from build123d import *

# Parameters (mm, degrees)
SKETCH1_R           = 15
BOSS_EXTRUDE1_DEPTH = 50
SKETCH2_R           = 1.5
BOSS_EXTRUDE2_DEPTH = 15
BOSS_EXTRUDE4_DEPTH = 3
SKETCH5_W           = 34
SKETCH5_H           = 3
BOSS_EXTRUDE5_DEPTH = 40
FILLET2_R           = 2
SKETCH6_R           = 30
BOSS_EXTRUDE6_DEPTH = 7
CUT_EXTRUDE1_DEPTH  = 7
SKETCH8_R           = 5
BOSS_EXTRUDE7_DEPTH = 5
SKETCH9_R           = 1.5
CUT_EXTRUDE2_DEPTH  = 5


with BuildPart() as part:
    # Sketch1 → Boss-Extrude1 (new body)
    with BuildSketch(Plane.XY):
        Circle(SKETCH1_R)
    extrude(amount=BOSS_EXTRUDE1_DEPTH)

    # Sketch2 → Boss-Extrude2 (add)
    with BuildSketch(Plane.XY.offset(50)):
        Circle(SKETCH2_R)
    extrude(amount=BOSS_EXTRUDE2_DEPTH)

    # Sketch4 → Boss-Extrude4 (add)
    with BuildSketch(Plane.XY.offset(50)):
        with BuildLine():
            Line((-17, 0), (-17, 30))
            Line((-17, 30), (17, 30))
            Line((17, 30), (17, 0))
            ThreePointArc((17, 0), (0, -17), (-17, 0))
        make_face()
    extrude(amount=BOSS_EXTRUDE4_DEPTH)

    # Sketch5 → Boss-Extrude5 (add)
    with BuildSketch(Plane(origin=(0, 0, 50), x_dir=(-1, 0, 0), z_dir=(0, 0, -1))):
        with Locations((0, 28.5)):
            Rectangle(SKETCH5_W, SKETCH5_H)
    extrude(amount=BOSS_EXTRUDE5_DEPTH)

    # Fillet2
    fillet2_edges = [part.edges().sort_by_distance(p)[0] for p in [
        (0, 30, 53),
        (0, 27, 50),
        (17, 28.5, 10),
        (-17, 28.5, 10),
    ]]
    fillet(fillet2_edges, radius=FILLET2_R)

    # Sketch6 → Boss-Extrude6 (add)
    with BuildSketch(Plane.XY.offset(65)):
        with Locations(Location((0, 0, 0), (0, 0, 180))):
            Circle(SKETCH6_R)
    extrude(amount=BOSS_EXTRUDE6_DEPTH)

    # Sketch7 → Cut-Extrude1 (cut)
    with BuildSketch(Plane.XY.offset(72)):
        with BuildLine():
            Line((0, 25), (0, 5))
            ThreePointArc((0, 5), (1.710100717, 4.698463104), (3.213938048, 3.830222216))
            Line((3.213938048, 3.830222216), (16.069690242, 19.151111078))
            ThreePointArc((16.069690242, 19.151111078), (8.550503583, 23.49231552), (0, 25))
        make_face()
        with BuildLine():
            Line((23.776412907, 7.725424859), (4.755282581, 1.545084972))
            ThreePointArc((4.755282581, 1.545084972), (4.996954135, -0.174497484), (4.635919273, -1.873032967))
            Line((4.635919273, -1.873032967), (23.179596364, -9.365164835))
            ThreePointArc((23.179596364, -9.365164835), (24.984770675, -0.872487418), (23.776412907, 7.725424859))
        make_face()
        with BuildLine():
            Line((14.694631307, -20.225424859), (2.938926261, -4.045084972))
            ThreePointArc((2.938926261, -4.045084972), (1.378186779, -4.80630848), (-0.348782369, -4.987820251))
            Line((-0.348782369, -4.987820251), (-1.743911844, -24.939101256))
            ThreePointArc((-1.743911844, -24.939101256), (6.890933895, -24.031542398), (14.694631307, -20.225424859))
        make_face()
        with BuildLine():
            Line((-14.694631307, -20.225424859), (-2.938926261, -4.045084972))
            ThreePointArc((-2.938926261, -4.045084972), (-4.145187863, -2.795964517), (-4.851478631, -1.209609478))
            Line((-4.851478631, -1.209609478), (-24.257393157, -6.04804739))
            ThreePointArc((-24.257393157, -6.04804739), (-20.725939314, -13.979822587), (-14.694631307, -20.225424859))
        make_face()
        with BuildLine():
            Line((-23.776412907, 7.725424859), (-4.755282581, 1.545084972))
            ThreePointArc((-4.755282581, 1.545084972), (-3.940053768, 3.078307377), (-2.649596321, 4.240240481))
            Line((-2.649596321, 4.240240481), (-13.247981606, 21.201202404))
            ThreePointArc((-13.247981606, 21.201202404), (-19.70026884, 15.391536883), (-23.776412907, 7.725424859))
        make_face()
    extrude(amount=-CUT_EXTRUDE1_DEPTH, mode=Mode.SUBTRACT)

    # Sketch8 → Boss-Extrude7 (add)
    with BuildSketch(Plane(origin=(0, 0, 65), x_dir=(-1, 0, 0), z_dir=(0, 0, -1))):
        with Locations(Location((0, 0, 0), (0, 0, 162))):
            Circle(SKETCH8_R)
    extrude(amount=BOSS_EXTRUDE7_DEPTH)

    # Sketch9 → Cut-Extrude2 (cut)
    with BuildSketch(Plane(origin=(0, 30, 0), x_dir=(1, 0, 0), z_dir=(0, 1, 0))):
        with Locations(Location((-12, -46, 0), (0, 0, 270))):
            Circle(SKETCH9_R)
        with Locations(Location((-12, -17, 0), (0, 0, 270))):
            Circle(SKETCH9_R)
        with Locations(Location((12, -46, 0), (0, 0, 270))):
            Circle(SKETCH9_R)
        with Locations(Location((12, -17, 0), (0, 0, 270))):
            Circle(SKETCH9_R)
    extrude(amount=-CUT_EXTRUDE2_DEPTH, mode=Mode.SUBTRACT)


solid = part.part
Could you check a few things on this model? Use its own coordinates, in mm. A direction names the side the tool comes from. Give positions to 0.01 mm unless a question says otherwise; leave off trailing zeros. Order: outer loops, then holes, each group sorted by start corner. A loop starts at its lowest first (then second) coordinate and runs counter-clockwise, first axis right, second up.
1. Suppose I cut it at D-D (z = 32). Write out the boundary of the cut face in (x, y), plus the area to 3 significant figures.
Answers below:
outline: (-17, 27) - (17, 27) - (17, 30) - (-17, 30) - close; circle Ø30 at (0, 0)
area: 809 mm2
2. Suppose I cut it at B-B (x = -6.5). Write out the boundary of the cut face in (y, z).
Answers below:
outline: (-29.29, 65) - (-8.95, 65) - (-8.95, 72) - (-29.29, 72) - close; (-15.71, 50) - (-13.52, 50) - (-13.52, 0) - (13.52, 0) - (13.52, 50) - (25, 50) arc R2 cw to (27, 48) - (27, 10) - (30, 10) - (30, 51) arc R2 ccw to (28, 53) - (-15.71, 53) - close; (-1.62, 65) - (2.11, 65) - (2.11, 72) - (-1.62, 72) - close; (10.4, 65) - (29.29, 65) - (29.29, 72) - (10.4, 72) - close
3. Suppose I cut it at A-A (z = 46). Write out the boundary of the cut face in (x, y).
Answers below:
outline: (-17, 27) - (-13.5, 27) - (-13.5, 30) - (-17, 30) - close; circle Ø30 at (0, 0); (-10.5, 27) - (10.5, 27) - (10.5, 30) - (-10.5, 30) - close; (13.5, 27) - (17, 27) - (17, 30) - (13.5, 30) - close
4. Suppose I cut it at C-C (y = -21.5). Write out the boundary of the cut face in (x, z), plus the area to 3 significant figures.
Answers below:
outline: (-20.92, 65) - (-1.5, 65) - (-1.5, 72) - (-20.92, 72) - close; (12.76, 65) - (20.92, 65) - (20.92, 72) - (12.76, 72) - close
area: 193 mm2
5. I need wall thicknesses on L1, parallel to X at y = 28.1, z = 46; L2, parallel to Y at x = 3, z = 68; L3, parallel to Y at x = 6.5, z = 42. Which ranges of each line are inside material? Lowest first, please.
Answers below:
L1: x = -17 to -13.5, -10.5 to 10.5, 13.5 to 17
L2: y = -29.85 to -24.82, -4.13 to 4, 24.82 to 29.85
L3: y = -13.52 to 13.52, 27 to 30
6. Which directions (+Z, -Z, +X, -X, +Y, -Y) give clear straight access to the entire face, cutting with the end or side of a thin tool? Please do faces 4 (the flat face through (-17, 27.2, 40.2)), 5 (the cylindrical face through (-20, 15, 69)), 6 (the flat face through (0, 29, 10)).
Answers below:
face 4: -Z, -X, +Y, -Y
face 5: +Z
face 6: -Z, +X, -X, +Y
7. For pin 1 (4 mm diameter, centred on x = -12, z = 46, fed in from -Y); pin 2 (24 mm diameter, centred on y = 9, z = 24.5, fed in from -X); pin 3 (2.5 mm diameter, centred on x = -12, z = 17, fed in from +Y), each with a flat end and sliding along its axis, tell me the tip position at first contact or that it passes through.
Answers below:
pin 1: stops at y = -11.18
pin 2: stops at x = -15
pin 3: stops at y = 10.46
8. Thinking about a two-plate mould opening in X: for faces 1 (the flat face through (0, 27, 29)), 2 (the cylindrical face through (16.43, 28.52, 10.6)), 3 (the flat face through (-1.037, -14.824, 68.549)), which applies, +X half, -X half, draft (parallel to the pull), parting line (faces both ways), or undercut?
Answers below:
face 1: draft
face 2: +X half
face 3: undercut
